The listing builds one solid part. Answer for the finished solid, in the listing's coordinates (mm). A direction names the side the tool comes from. Round coordinates to 2 decimals unless told otherwise and drop trailing zeros. Order: outer loops, then holes, each group sorted by start corner. A loop starts at its lowest first (then second) coordinate and runs counter-clockwise, first axis right, second up. Notation, with made-up numbers: (31, 72) -> (73, 72) arc R16 ccw to (73, 97) -> close; hole circle Ø2 at (17.25, -1.5). An arc over 180 degrees is marked (long way). Return JSON: item names as keys, results as strings. Group by question number.
(1) Which of the six approach directions +Z, -Z, +X, -X, +Y, -Y give full straight-line access (tool end or side, diameter ignored) to faces 1 (the face through (-25.799, 30.273, -12.878)), 2 (the face through (-23.92, -7.85, -17))?
(2) Each of these flat-tipped pins is pushed along its axis until it touches: pin 1 (3 mm diameter, centred on y = 17, z = -16, fed in from +X); pin 2 (8 mm diameter, centred on y = 10.5, z = -13, fed in from -X); pin 3 (4 mm diameter, centred on x = -27.5, z = -21, fed in from +Y); pin 4 (1.5 mm diameter, centred on y = 9.5, z = -14.5, fed in from -X). Where does it stop, or does it pass through?
(3) The part is cut by section D-D (z = -31). Determine the outline of the cut face in (x, y), plus the area to 3 significant figures.
(4) The part is cut by section A-A (y = 17). Determine the outline of the cut face in (x, z).
(5) The part is cut by section B-B (x = -28). Determine the outline of the cut face in (y, z), plus the area to 3 significant figures.
(6) Consider line 1 (Z direction, x = -31, y = 21); line 2 (X direction, y = 16.5, z = -12.5); line 3 (X direction, y = 17, z = -21). Determine where each line is inside the solid, lowest interval first. Write a range as [from, to].
(7) The part is cut by section C-C (z = -16.5). Determine the outline of the cut face in (x, y).
from build123d import *

# Parameters (mm, degrees)
F0_R      = 24.311566
F1_DEPTH  = 33.528
F2_R      = 24.311566
F2_R_2    = 6.595336
F1_FACE_R = 24.311566
F3_DEPTH  = 25.4
F4_R      = 24.311566
F4_R_2    = 10.101211
F5_DEPTH  = 25.4


with BuildPart() as f1:
    # F0 (on Top) → F1 (new body)
    with BuildSketch(Plane.XY):
        with Locations((-18.654427, 15.885411)):
            Circle(F0_R)
    extrude(amount=-F1_DEPTH)

    # F2 (on face) + F1_face (on face) → F3 (cut)
    with BuildSketch(Plane.XY):
        with Locations((-18.654427, 15.885411)):
            Circle(F2_R)
        with Locations((-23.900984, 19.966066)):
            Circle(F2_R_2, mode=Mode.SUBTRACT)
        with Locations((-23.900984, 19.966066)):
            Circle(F2_R_2)
    with BuildSketch(Plane(origin=(-18.654427, 15.885411, 0), x_dir=(1, 0, 0), z_dir=(0, 0, 1))):
        Circle(F1_FACE_R)
    extrude(amount=-F3_DEPTH, mode=Mode.SUBTRACT)

    # F4 (on face) → F5 (join)
    with BuildSketch(Plane.XY.offset(-25.4)):
        with Locations((-18.654427, 15.885411)):
            Circle(F4_R)
        with Locations((-24.483934, 20.257542)):
            Circle(F4_R_2, mode=Mode.SUBTRACT)
    extrude(amount=F5_DEPTH)


solid = f1.part
Answer below:
{
 "1": {"face 1": "+Z", "face 2": "+Z, -Z"},
 "2": {"pin 1": "stops at x = 5.66", "pin 2": "stops at x = -42.93", "pin 3": "stops at y = 39.21", "pin 4": "stops at x = -42.3"},
 "3": {"outline": "circle Ø48.62 at (-18.65, 15.89)", "area": "1,860 mm²"},
 "4": {"outline": "(-42.94, -33.53) -> (5.63, -33.53) -> (5.63, 0) -> (-14.92, 0) -> (-14.92, -25.4) -> (-34.05, -25.4) -> (-34.05, 0) -> (-42.94, 0) -> close"},
 "5": {"outline": "(-6.56, -33.53) -> (38.33, -33.53) -> (38.33, 0) -> (29.73, 0) -> (29.73, -25.4) -> (10.79, -25.4) -> (10.79, 0) -> (-6.56, 0) -> close", "area": "1,020 mm²"},
 "6": {"line 1": "z = [-33.53, -25.4]", "line 2": "x = [-42.96, -33.86], [-15.11, 5.65]", "line 3": "x = [-42.94, -34.05], [-14.92, 5.63]"},
 "7": {"outline": "circle Ø48.62 at (-18.65, 15.89); hole circle Ø20.2 at (-24.48, 20.26)"}
}
